Design review of the part built by this model. Coordinates are the model's own, in mm. Face numbers are marked on the shaded views. A direction names the side the tool comes from. Coordinates: 2 decimals unless noted, no trailing zeros. Write each loop counter-clockwise with the first axis right and the second up, starting at its lowest first coordinate (ties: lowest second). Pieces come first, ordered by that corner, then holes. Notation, with made-up numbers: M -32.5,2 L -0.5,2 A27 ccw -0.5,26 Z; hole C 24.5,26 d9. An arc over 180 degrees is marked long. Write item = value, one per line.
Autodesk Inventor part; units mm, degrees
ref_plane "YZ Plane" through (0, 0, 0) normal (1, 0, 0) x (0, 1, 0)
ref_plane "XZ Plane" through (0, 0, 0) normal (0, 1, 0) x (-1, 0, 0)
ref_plane "XY Plane" through (0, 0, 0) normal (0, 0, 1) x (1, 0, 0)
sketch "Sketch1" plane through (0, 0, 0) normal (0, 0, 1) x (1, 0, 0)
  circle A0 centre (0, 0) radius 37.5
  circle A1 centre (0, 25) radius 2.5
  circle A2 centre (0, 0) radius 25 construction
  circle A3 centre (-21.6506, 12.5) radius 2.5
  circle A4 centre (-21.6506, -12.5) radius 2.5
  circle A5 centre (0, -25) radius 2.5
  circle A6 centre (21.6506, -12.5) radius 2.5
  circle A7 centre (21.6506, 12.5) radius 2.5
  circle A8 centre (0, 0) radius 2.5
  dimension "d2" = 50
  dimension "d0" = 75
  dimension "d1" = 5
  dimension "d5" = 360
  dimension "d7" = 5
extrude "Extrusion1" add sketch "Sketch1" along normal blind 10
sketch "Sketch4" plane through (0, 0, 10) normal (0, 0, 1) x (1, 0, 0)
  circle A0 centre (0, 0) radius 2.5
  circle A1 centre (21.6506, 12.5) radius 2.5
  circle A2 centre (21.6506, -12.5) radius 2.5
  circle A3 centre (0, -25) radius 2.5
  circle A4 centre (-21.6506, -12.5) radius 2.5
  circle A5 centre (-21.6506, 12.5) radius 2.5
  circle A6 centre (0, 25) radius 2.5
  circle A7 centre (0, 0) radius 37.5
  circle A8 centre (0, 25) radius 6
  circle A9 centre (-21.6506, 12.5) radius 6
  circle A10 centre (-21.6506, -12.5) radius 6
  circle A11 centre (0, -25) radius 6
  circle A12 centre (21.6506, -12.5) radius 6
  circle A13 centre (21.6506, 12.5) radius 6
  dimension "d17" = 12
  dimension "d20" = 360
extrude "Extrusion4" cut sketch "Sketch4" against normal blind 5 contours A8 | A9 | A10 | A11 | A12 | A13
sketch "Sketch5" plane through (0, 0, 0) normal (0, 0, -1) x (-1, 0, 0)
  circle A0 centre (0, 0) radius 2.5
  circle A1 centre (0, 0) radius 8.5
  dimension "d24" = 17
extrude "Extrusion5" cut sketch "Sketch5" against normal blind 5
sketch "Sketch6" plane through (0, 0, 10) normal (0, 0, 1) x (1, 0, 0)
  circle A0 centre (0, 0) radius 2.5
  circle A1 centre (0, 0) radius 14
  circle A2 centre (0, 0) radius 17.5
  dimension "d35" = 35
  dimension "d36" = 28
extrude "Extrusion6" add sketch "Sketch6" along normal blind 10 contours A2
sketch "Sketch7" plane through (0, 0, 20) normal (0, 0, 1) x (1, 0, 0)
  circle A0 centre (0, 0) radius 6
  circle A1 centre (0, 0) radius 2.5
  circle A2 centre (0, 0) radius 17.5
  circle A3 centre (0, 0) radius 17.5
  dimension "d40" = 12
extrude "Extrusion7" add sketch "Sketch7" against normal blind 4 contours A2
sketch "Sketch8" plane through (0, 0, 20) normal (0, 0, 1) x (1, 0, 0)
  circle A0 centre (0, 0) radius 37.5
  line L0 (0, -37.5) -> (37.5, -37.5)
  line L1 (37.5, -37.5) -> (37.5, 37.5)
  line L2 (37.5, 37.5) -> (0, 37.5)
  line L3 (0, 37.5) -> (0, -37.5)
  point P0 (37.5, 0)
extrude "Extrusion8" cut sketch "Sketch8" against normal through all contours A0 L3 | L1 L0 A0 | A0 L2 L1 picked at (9.7729, 7.7936)
sketch "Sketch9" plane through (0, 0, 5) normal (0, 0, -1) x (-1, 0, 0)
  arc A0 (0, 14) -> (0, -14) centre (0, 0) ccw
  circle A1 centre (0, 0) radius 8.5 construction
  arc A2 (0, -14) -> (0, 14) centre (0, 0) ccw
  line L0 (0, 14) -> (-0.0015, 8.5)
  line L1 (0, -14) -> (0, -8.5)
  line L2 (0, -6) -> (0, -14)
  arc A3 (0, -8.5) -> (-0.0015, 8.5) centre (0, 0) ccw
  line L3 (0, 8.5) -> (0, 2.5)
  dimension "d39" = 17
extrude "Extrusion9" cut sketch "Sketch9" against normal blind 5 contours L0 A3 L1 A0
properties part number "BA008" material "ABS Plastic"
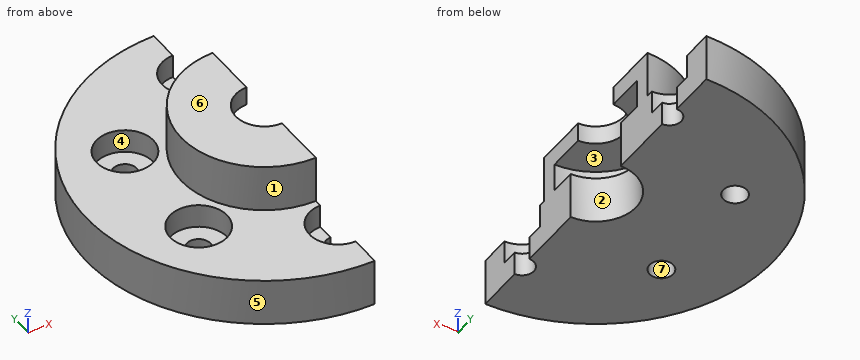
Q1. Consider section A-A, the plane z = 8. State the section outline as (x, y) points, and give its area (3 significant figures).
Check result:
outline = M 0,-37.5 L 0,-31 A6 cw 0,-19 L 0,-8.5 A8.5 cw 0,8.5 L 0,19 A6 cw 0,31 L 0,37.5 A37.5 ccw Z; hole C -21.65,-12.5 d12; hole C -21.65,12.5 d12
area = 1,760 mm²
Q2. Consider section B-B, the plane y = 0. State the section outline as (x, z) points.
Check result:
outline = M -37.5,0 L -8.5,0 L -8.5,10 L -14,10 L -14,16 L -6,16 L -6,20 L -17.5,20 L -17.5,10 L -37.5,10 Z
Q3. Consider section C-C, the plane y = -12.5. State the section outline as (x, z) points.
Check result:
outline = M -35.36,0 L -24.15,0 L -24.15,5 L -27.65,5 L -27.65,10 L -35.36,10 Z; M -19.15,0 L 0,0 L 0,10 L -6.3,10 L -6.3,16 L 0,16 L 0,20 L -12.25,20 L -12.25,10 L -15.65,10 L -15.65,5 L -19.15,5 Z
Q4. The part is to be moulded in two halves that separate along Y. For the marked faces 5, 6 and 7, say which applies: +Y half, -Y half, draft (parallel to the pull), parting line (faces both ways), or undercut.
Check result:
face_5 = parting line
face_6 = draft
face_7 = undercut
Q5. For P1, Ø8, axis at x = -17, y = -10, coming from the -Z side; P2, Ø5, axis at y = 26, z = 7, coming from the -X side; P3, Ø1.5, axis at y = -23, z = 9, coming from the -X side; P4, Ø3, axis at x = -21.65, y = -12.5, coming from the -Z side, all flat-tipped, find the tip position at first contact; note any pin that passes through.
Check result:
P1 = 0
P2 = -29.22
P3 = -30.19
P4 = through
Q6. Machinability: for the marked faces 1, 2, 3 and 4, which of the approach directions +Z, -Z, +X, -X, +Y, -Y give a long, thin tool a straight path to every point of the face, cutting with its end or side? Answer none if there is none.
Check result:
face_1 = +Z, -X
face_2 = -Z, +X
face_3 = +X
face_4 = +Z
Q7. Consider section D-D, the plane z = 13. State the section outline as (x, y) points, and give its area (3 significant figures).
Check result:
outline = M 0,-17.5 L 0,-14 A14 cw 0,14 L 0,17.5 A17.5 ccw Z
area = 173 mm²
Q8. Wall thickness on line 1 (Y direction, x = -10.5, z = 18); line 2 (Z direction, x = -9, y = -3); line 3 (Z direction, x = -14, y = -25): over which ranges is each line inside the solid? List them lowest first.
Check result:
line_1 = -14 to 14
line_2 = 0 to 10, 16 to 20
line_3 = 0 to 10
